Answer from the drawing. Dimensions are ordinates in mm from the lowest x, y and z of the part. A direction names the side the tool comes from. Coordinates: 2 decimals unless noted, no trailing zeros. Order: outer loops, then holes, each group sorted by start corner. A loop starts at its lowest first (then second) coordinate and runs counter-clockwise, first axis right, second up.
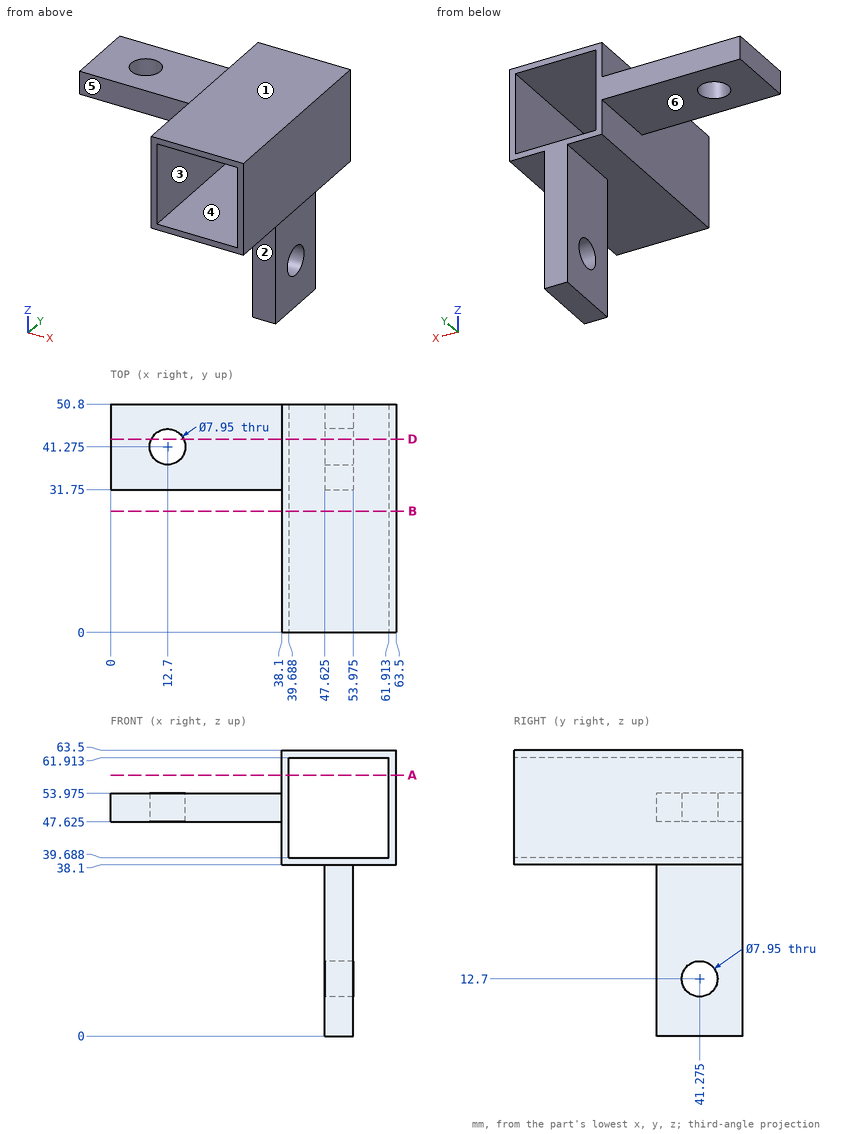
1. The part is cut by section A-A (z = 58). Determine the outline of the cut face in (x, y).
2. For the marked faces 4, 5 and 6, determine the directions among +Z, -Z, +X, -X, +Y, -Y from which every point of the face is accessible in a straight line to the end or side of a thin tool.
3. The part is cut by section D-D (y = 43). Determine the outline of the cut face in (x, z) (1 decimal).
4. The part is cut by section B-B (y = 27). Determine the outline of the cut face in (x, z), plus the area to 3 significant figures.
5. Flat-ended cylindrical pins translate along their axes: pin 1 (2 mm diameter, centred on x = 39, y = 42, fed in from -Z); pin 2 (5 mm diameter, centred on y = 40, z = 26.5, fed in from -X) (1 decimal); pin 3 (5 mm diameter, centred on x = 20, z = 51, fed in from -Y); pin 4 (20.5 mm diameter, centred on x = 53, y = 26.5, fed in from -Z). Find the tip coordinate at first contact, or state that the pin passes through.
6. Consider probe 1 along Y at (x, z) = (49.5, 22); probe 2 along X at (y, z) = (9.5, 52). Determine where each line is inside the solid, lowest interval first.
7. The mould has two halves that part along Z. Classify the marked faces 1, 2 and 3: released by +Z, released by -Z, zero draft, split by the parting line, or undercut.
Worked out:
1. outline: (38.1, 0) - (39.69, 0) - (39.69, 50.8) - (38.1, 50.8) - close; (61.91, 0) - (63.5, 0) - (63.5, 50.8) - (61.91, 50.8) - close
2. face 4: +Y, -Y
2. face 5: +Z, -Z, -X, -Y
2. face 6: -Z, -X, +Y, -Y
3. outline: (0, 47.6) - (9.1, 47.6) - (9.1, 54) - (0, 54) - close; (16.3, 47.6) - (38.1, 47.6) - (38.1, 38.1) - (47.6, 38.1) - (47.6, 16.3) - (54, 16.3) - (54, 38.1) - (63.5, 38.1) - (63.5, 63.5) - (38.1, 63.5) - (38.1, 54) - (16.3, 54) - close; (47.6, 0) - (54, 0) - (54, 9.1) - (47.6, 9.1) - close; hole (39.7, 39.7) - (61.9, 39.7) - (61.9, 61.9) - (39.7, 61.9) - close
4. outline: (38.1, 38.1) - (63.5, 38.1) - (63.5, 63.5) - (38.1, 63.5) - close; hole (39.69, 39.69) - (61.91, 39.69) - (61.91, 61.91) - (39.69, 61.91) - close
4. area: 151 mm2
5. pin 1: stops at z = 38.1
5. pin 2: stops at x = 47.6
5. pin 3: stops at y = 31.75
5. pin 4: stops at z = 0
6. probe 1: y = 31.75 to 50.8
6. probe 2: x = 38.1 to 39.69, 61.91 to 63.5
7. face 1: released by +Z
7. face 2: zero draft
7. face 3: undercut
